Geometry check sheet. Reference: the model listing, model coordinates, mm. Give positions to 0.01 mm unless a question says otherwise; leave off trailing zeros. Loops run counter-clockwise (first coordinate to the right, second up) from the corner with the lowest first, then second, coordinate; pieces in that order, holes last.
1. Cross-section at B-B, the plane x = 4. Record the cut outline in (y, z).
2. Cross-section at A-A, the plane z = -14.5. Record the cut outline in (x, y) (3 decimals), plus the area to 3 significant figures.
3. Cross-section at C-C, the plane y = 4.75. Record the cut outline in (x, z), plus the area to 3 significant figures.
4. Go/stop test with flat-tipped pins: pin 1 Ø0.7 at (y, z) = (0, 35.5) entering from -X; pin 2 Ø0.7 at (y, z) = (0, 36) entering from +X; pin 3 Ø1 at (x, z) = (2, -2.5) entering from -Y. Record where each tip stops, or that it passes through.
5. Material ranges on L1, parallel to X at y = -0.25, z = 23.5; L2, parallel to Y at x = -2, z = 14, recorded low to high.
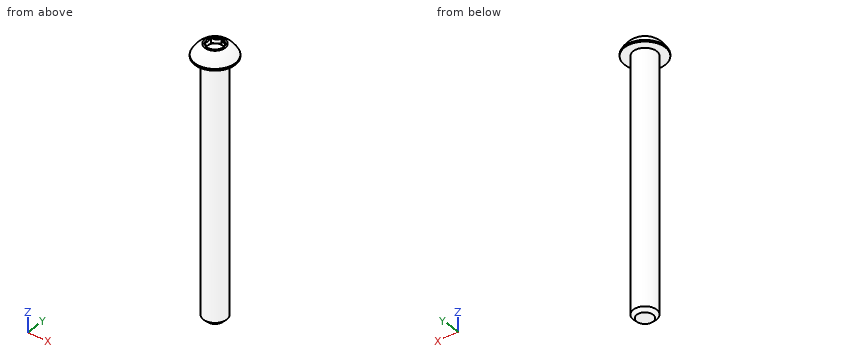
from build123d import *

# Parameters (mm, degrees)
CUT_EXTRUDE1_START = 35.26028
CUT_EXTRUDE1_DEPTH = 2.34112
SKETCH4_R          = 2.291358881
CUT_EXTRUDE2_DEPTH = 1.34112
CUT_EXTRUDE2_DRAFT = -45


with BuildPart() as part:
    # Sketch2 → Revolve1 (revolve)
    with BuildSketch(Plane(origin=(0, 0, 0), x_dir=(0, 0, -1), z_dir=(1, 0, 0))):
        with BuildLine():
            Line((-36.6014, 1.984375), (-36.6014, 2.778125))
            ThreePointArc((-36.6014, 2.778125), (-35.386122602, 4.40912482), (-33.702171429, 5.5499))
            Line((-33.702171429, 5.5499), (-33.2486, 5.5499))
            Line((-33.2486, 5.5499), (-33.2486, 3.175))
            Line((-33.2486, 3.175), (35.6489, 3.175))
            Line((35.6489, 3.175), (36.6014, 2.2225))
            Line((36.6014, 2.2225), (36.6014, 0))
            Line((36.6014, 0), (-34.11460056, 0))
            Line((-34.11460056, 0), (-35.26028, 1.984375))
            Line((-35.26028, 1.984375), (-36.6014, 1.984375))
        make_face()
    revolve(axis=Axis((0, 0, 36.6014), (0, 0, -1)))

    # Sketch3 → Cut-Extrude1 (cut, through all)
    with BuildSketch(Plane.XY.offset(CUT_EXTRUDE1_START)):
        Polygon((0, 2.291358881), (-1.984375, 1.14567944), (-1.984375, -1.14567944), (0, -2.291358881), (1.984375, -1.14567944), (1.984375, 1.14567944), align=None)
    extrude(amount=CUT_EXTRUDE1_DEPTH, mode=Mode.SUBTRACT)


with BuildPart() as cut_extrude2_tool:
    # Sketch4 → Cut-Extrude2 (with draft: the straight prism first)
    with BuildSketch(Plane.XY.offset(36.6014)):
        Circle(SKETCH4_R)
    extrude(amount=-CUT_EXTRUDE2_DEPTH)
    # Cut-Extrude2: the draft: its side faces are tilted about the plane it starts from
    cut_extrude2_sides = [cut_extrude2_tool.faces().sort_by_distance(p)[0] for p in [
        (-2.291358881, 0, 35.93084),
    ]]
    draft(cut_extrude2_sides, Plane.XY.offset(36.6014), CUT_EXTRUDE2_DRAFT)


with BuildPart() as part_1:
    add(part.part)

    # Cut-Extrude2: cut by cut_extrude2_tool
    add(cut_extrude2_tool.part, mode=Mode.SUBTRACT)


solid = part_1.part
Result:
1. outline: (-3.85, 33.25) - (3.85, 33.25) - (3.85, 33.7) arc R4.61 ccw to (-3.85, 33.7) - close
2. outline: circle Ø6.35 at (0, 0)
2. area: 31.7 mm2
3. outline: (-2.87, 33.25) - (2.87, 33.25) - (2.87, 33.7) arc R3.83 ccw to (-2.87, 33.7) - close
3. area: 7.76 mm2
4. pin 1: stops at x = -4.62
4. pin 2: stops at x = 4.14
4. pin 3: stops at y = -2.8
5. L1: x = -3.17 to 3.17
5. L2: y = -2.47 to 2.47
